from build123d import *

# Parameters (mm, degrees)
F1_DEPTH = 304.8
F2_DEPTH = 368.3
F3_R     = 127
F4_DEPTH = 596.9
F5_R     = 127
F6_DEPTH = 190.501


with BuildPart() as f1:
    # F0 (on Front) → F1 (new body, symmetric)
    with BuildSketch(Plane.XZ):
        with BuildLine():
            Line((457.2, 0), (508, 0))
            ThreePointArc((508, 0), (359.210245, 359.210245), (0, 508))
            Line((0, 508), (0, 457.2))
            ThreePointArc((0, 457.2), (323.28922, 323.28922), (457.2, 0))
        make_face()
        with BuildLine():
            Line((508, -406.4), (508, 0))
            Line((508, 0), (457.2, 0))
            ThreePointArc((457.2, 0), (323.28922, -323.28922), (0, -457.2))
            ThreePointArc((0, -457.2), (-323.28922, -323.28922), (-457.2, 0))
            Line((-457.2, 0), (-508, 0))
            Line((-508, 0), (-508, -406.4))
            Line((-508, -406.4), (-1016, -406.4))
            Line((-1016, -406.4), (-1016, -596.9))
            Line((-1016, -596.9), (1016, -596.9))
            Line((1016, -596.9), (1016, -406.4))
            Line((1016, -406.4), (508, -406.4))
        make_face()
        with BuildLine():
            Line((0, 457.2), (0, 508))
            ThreePointArc((0, 508), (-359.210245, 359.210245), (-508, 0))
            Line((-508, 0), (-457.2, 0))
            ThreePointArc((-457.2, 0), (-323.28922, 323.28922), (0, 457.2))
        make_face()
    extrude(amount=F1_DEPTH, both=True)

    # F0 (on Front) → F2 (join, symmetric)
    with BuildSketch(Plane.XZ):
        with BuildLine():
            ThreePointArc((-457.2, 0), (-323.28922, -323.28922), (0, -457.2))
            Line((0, -457.2), (0, -355.6))
            ThreePointArc((0, -355.6), (-251.447171, -251.447171), (-355.6, 0))
            Line((-355.6, 0), (-457.2, 0))
        make_face()
        with BuildLine():
            ThreePointArc((0, -457.2), (323.28922, -323.28922), (457.2, 0))
            Line((457.2, 0), (355.6, 0))
            ThreePointArc((355.6, 0), (251.447171, -251.447171), (0, -355.6))
            Line((0, -355.6), (0, -457.2))
        make_face()
        with BuildLine():
            Line((355.6, 0), (457.2, 0))
            ThreePointArc((457.2, 0), (323.28922, 323.28922), (0, 457.2))
            Line((0, 457.2), (0, 355.6))
            ThreePointArc((0, 355.6), (251.447171, 251.447171), (355.6, 0))
        make_face()
        with BuildLine():
            Line((0, 355.6), (0, 457.2))
            ThreePointArc((0, 457.2), (-323.28922, 323.28922), (-457.2, 0))
            Line((-457.2, 0), (-355.6, 0))
            ThreePointArc((-355.6, 0), (-251.447171, 251.447171), (0, 355.6))
        make_face()
    extrude(amount=F2_DEPTH, both=True)

    # F3 (on face) → F4 (cut)
    with BuildSketch(Plane.XY.offset(-406.4)):
        with Locations((-762, 0)):
            Circle(F3_R)
        with BuildLine():
            ThreePointArc((-969.202229, -304.8), (-1004.232409, -154.185825), (-1016, -5e-06))
            Line((-1016, -5e-06), (-1016, -304.8))
            Line((-1016, -304.8), (-969.202229, -304.8))
        make_face()
        with BuildLine():
            ThreePointArc((-1016, -5e-06), (-1004.23241, 154.18582), (-969.202229, 304.8))
            Line((-969.202229, 304.8), (-1016, 304.8))
            Line((-1016, 304.8), (-1016, -5e-06))
        make_face()
    extrude(amount=-F4_DEPTH, mode=Mode.SUBTRACT)

    # F5 (on face) → F6 (cut, through all)
    with BuildSketch(Plane.XY.offset(-406.4)):
        with BuildLine():
            ThreePointArc((969.202229, 304.8), (1004.232409, 154.185822), (1016, 0))
            Line((1016, 0), (1016, 304.8))
            Line((1016, 304.8), (969.202229, 304.8))
        make_face()
        with BuildLine():
            ThreePointArc((1016, 0), (1004.232409, -154.185822), (969.202229, -304.8))
            Line((969.202229, -304.8), (1016, -304.8))
            Line((1016, -304.8), (1016, 0))
        make_face()
        with Locations((762, 0)):
            Circle(F5_R)
    extrude(amount=-F6_DEPTH, mode=Mode.SUBTRACT)


solid = f1.part
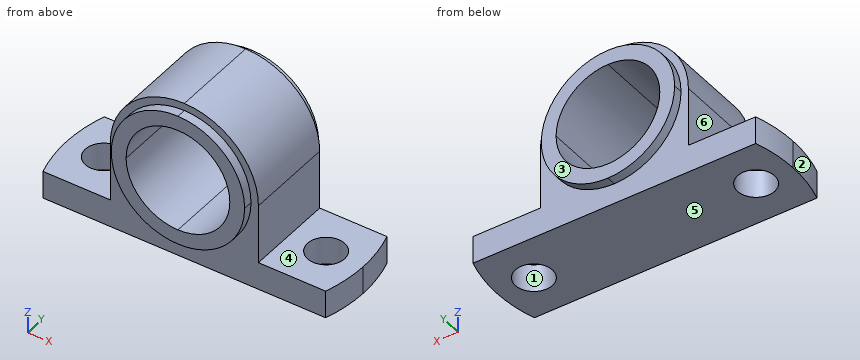
Input: part model. Units: mm. Frame: model coordinates. Face numbers are marked on the shaded views. A direction names the side the tool comes from. Coordinates: 2 decimals unless noted, no trailing zeros. Order: outer loops, then holes, each group sorted by start corner. A loop starts at its lowest first (then second) coordinate and runs counter-clockwise, first axis right, second up. Notation, with made-up numbers: M 20.5,-28.75 L 63.5,-28.75 A33 cw 63.5,5.25 Z; hole C 8.5,-26.75 d3. An arc over 180 degrees is marked long. Write item = value, one per line. Start each with the question number.
(1) First-contact query: P1, Ø2, axis at x = 317, y = -190.5, coming from the +Z side; P2, Ø1.5, axis at x = -752.5, y = 161.5, coming from the +Z side; P3, Ø3, axis at y = -112, z = -377.5, coming from the +X side. Flat tips, straight axial feed; report the tip coordinate or a pass-through.
(2) Line query: line 1 along Y through (x, z) = (-762, -474); line 2 along X through (y, z) = (86.5, -421); line 3 along Z through (x, y) = (-540.5, -302.5). Output: solid intervals per line, ascending. Write a range as [from, to].
(3) Pull-direction query (X, two-part tool) for the marked faces 1, 2 and 3; classes: released by +X, released by -X, zero draft, split by the parting line, or undercut.
(4) Section C-C on z = 112. Output: boundary loops of the cut face in (x, y).
(5) Reachability of the marked faces 4, 5 and 6 from +Z, -Z, +X, -X, +Y, -Y: full face, straight path, thin tool, end or side. Return the list, or none.
(6) Section B-B on y = -51. Output: boundary loops of the cut face in (x, z).
(7) Section D-D on y = 284. Output: boundary loops of the cut face in (x, z), and give its area (3 significant figures).
(8) Section A-A on x = 762. Output: boundary loops of the cut face in (y, z).
Result set:
q1.P1 = 397.75
q1.P2 = -406.4
q1.P3 = 508
q2.line_1 = [-304.8, -127], [127, 304.8]
q2.line_2 = [-1012.31, -854.99], [-669.01, 669.01], [854.99, 1012.31]
q2.line_3 = [-596.9, -406.4]
q3.face_1 = undercut
q3.face_2 = released by -X
q3.face_3 = zero draft
q4.outline = M -495.5,-304.8 L -443.27,-304.8 L -443.27,-368.3 L -337.5,-368.3 L -337.5,368.3 L -443.27,368.3 L -443.27,304.8 L -495.5,304.8 Z; M 337.5,-368.3 L 443.27,-368.3 L 443.27,-304.8 L 495.5,-304.8 L 495.5,304.8 L 443.27,304.8 L 443.27,368.3 L 337.5,368.3 Z
q5.face_4 = +Z, +X, +Y, -Y
q5.face_5 = -Z, +X, -X, +Y, -Y
q5.face_6 = +Z, -X, +Y, -Y
q6.outline = M -1014.72,-596.9 L -878.31,-596.9 L -878.31,-406.4 L -1014.72,-406.4 Z; M -645.69,-596.9 L 645.69,-596.9 L 645.69,-406.4 L 508,-406.4 L 508,0 A508 ccw 0,508 A508 ccw -508,0 L -508,-406.4 L -645.69,-406.4 Z; M 878.31,-596.9 L 1014.72,-596.9 L 1014.72,-406.4 L 878.31,-406.4 Z; hole M -355.6,0 A355.6 ccw 0,-355.6 A355.6 ccw 355.6,0 A355.6 ccw 0,355.6 A355.6 ccw Z
q7.outline = M -975.5,-596.9 L 975.5,-596.9 L 975.5,-406.4 L 508,-406.4 L 508,0 A508 ccw 0,508 A508 ccw -508,0 L -508,-406.4 L -975.5,-406.4 Z; hole M -355.6,0 A355.6 ccw 0,-355.6 A355.6 ccw 355.6,0 A355.6 ccw 0,355.6 A355.6 ccw Z
q7.area = 793,000 mm²
q8.outline = M -304.8,-596.9 L -127,-596.9 L -127,-406.4 L -304.8,-406.4 Z; M 127,-596.9 L 304.8,-596.9 L 304.8,-406.4 L 127,-406.4 Z
